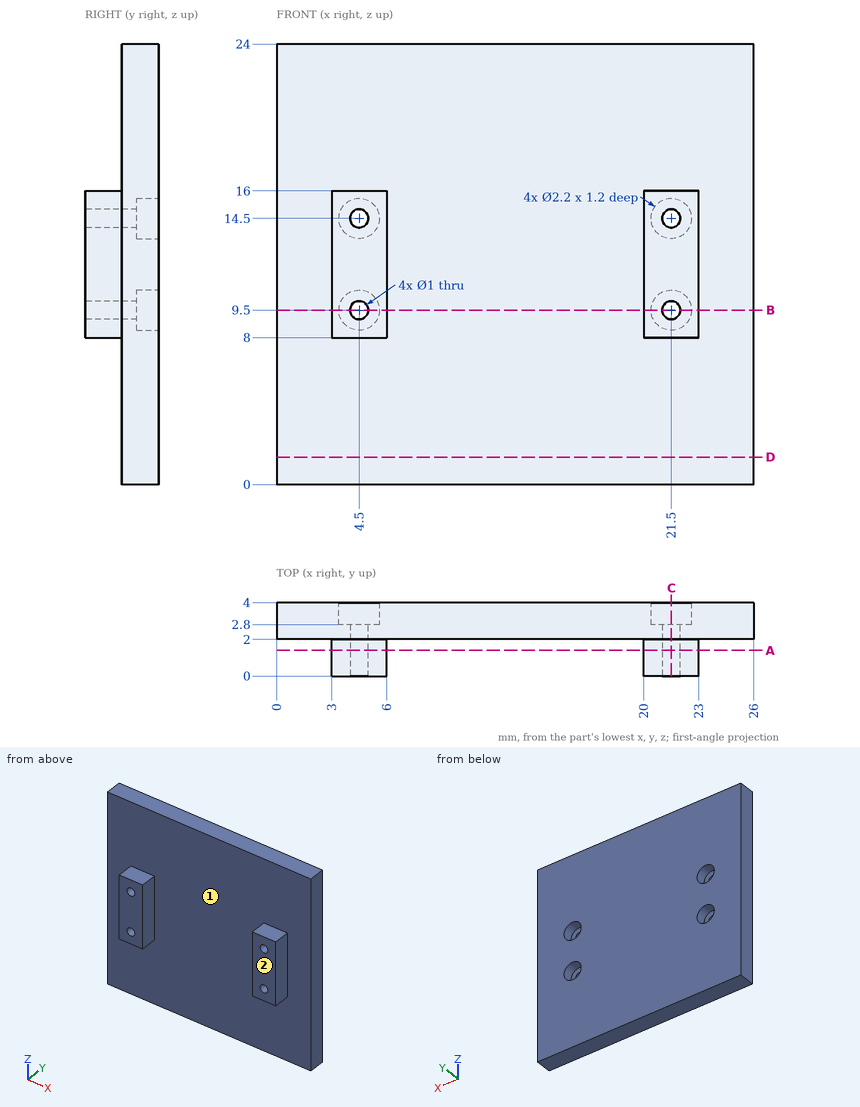
Geometry check sheet. Reference: drawing and pictorial views, mm from the part's lowest x, y, z. Give positions to 0.01 mm unless a question says otherwise; leave off trailing zeros. Write each loop counter-clockwise with the first axis right and the second up, starting at its lowest first coordinate (ties: lowest second). Pieces come first, ordered by that corner, then holes. Notation, with made-up numbers: (66, 32) - (99, 32) arc R13 cw to (99, 57) - close; hole circle Ø10 at (-6, -9.75). An arc over 180 degrees is marked (long way). Use a Markdown table: item, result.
Q1. Go/stop test with flat-tipped pins: P1, Ø1.8, axis at x = 4.5, z = 9.5, coming from the +Y side; P2, Ø1, axis at y = 1, z = 11.5, coming from the -X side; P3, Ø1, axis at x = 4, y = 1, coming from the +Z side. Record where each tip stops, or that it passes through.
Computed:
| item | result |
|---|---|
| P1 | stops at y = 2.8 |
| P2 | stops at x = 3 |
| P3 | stops at z = 16 |
Q2. Section check B-B, the plane z = 9.5. Enter the section's corners in (x, y).
Computed:
| item | result |
|---|---|
| outline | (0, 2) - (3, 2) - (3, 0) - (4, 0) - (4, 2.8) - (3.4, 2.8) - (3.4, 4) - (0, 4) - close; (5, 0) - (6, 0) - (6, 2) - (20, 2) - (20, 0) - (21, 0) - (21, 2.8) - (20.4, 2.8) - (20.4, 4) - (5.6, 4) - (5.6, 2.8) - (5, 2.8) - close; (22, 0) - (23, 0) - (23, 2) - (26, 2) - (26, 4) - (22.6, 4) - (22.6, 2.8) - (22, 2.8) - close |
Q3. Draft check along X on the marked faces 1 and 2. Enter one of: pulls with the +X half, pulls with the -X half, needs draft (parallel to the pull), parting line crosses it, or undercut.
Computed:
| item | result |
|---|---|
| face 1 | undercut |
| face 2 | needs draft |
Q4. Section check A-A, the plane y = 1.4. Enter the section's corners in (x, z).
Computed:
| item | result |
|---|---|
| outline | (3, 8) - (6, 8) - (6, 16) - (3, 16) - close; (20, 8) - (23, 8) - (23, 16) - (20, 16) - close; hole circle Ø1 at (4.5, 9.5); hole circle Ø1 at (4.5, 14.5); hole circle Ø1 at (21.5, 9.5); hole circle Ø1 at (21.5, 14.5) |
Q5. Section check D-D, the plane z = 1.5. Enter the section's corners in (x, y), then the cut area to 3 significant figures.
Computed:
| item | result |
|---|---|
| outline | (0, 2) - (26, 2) - (26, 4) - (0, 4) - close |
| area | 52.0 mm² |
Q6. Thickness scan on L1, parallel to Z at x = 21.5, y = 3.2; L2, parallel to X at y = 0.7, z = 14.5; L3, parallel to X at y = 1.3, z = 10.5. Record the ranges inside material, lowest first. Write a range as [from, to].
Computed:
| item | result |
|---|---|
| L1 | z = [0, 8.4], [10.6, 13.4], [15.6, 24] |
| L2 | x = [3, 4], [5, 6], [20, 21], [22, 23] |
| L3 | x = [3, 6], [20, 23] |
Q7. Section check C-C, the plane x = 21.5. Enter the section's corners in (y, z).
Computed:
| item | result |
|---|---|
| outline | (0, 8) - (2, 8) - (2, 0) - (4, 0) - (4, 8.4) - (2.8, 8.4) - (2.8, 9) - (0, 9) - close; (0, 10) - (2.8, 10) - (2.8, 10.6) - (4, 10.6) - (4, 13.4) - (2.8, 13.4) - (2.8, 14) - (0, 14) - close; (0, 15) - (2.8, 15) - (2.8, 15.6) - (4, 15.6) - (4, 24) - (2, 24) - (2, 16) - (0, 16) - close |
